Autodesk Inventor part; units mm, degrees
ref_plane "YZ Plane" through (0, 0, 0) normal (1, 0, 0) x (0, 1, 0)
ref_plane "XZ Plane" through (0, 0, 0) normal (0, 1, 0) x (-1, 0, 0)
ref_plane "XY Plane" through (0, 0, 0) normal (0, 0, 1) x (1, 0, 0)
sketch "Sketch1" plane through (0, 0, 0) normal (0, 0, 1) x (1, 0, 0)
  line L0 (-47.9977, 34.7826) -> (52.0023, 34.7826)
  line L1 (52.0023, 34.7826) -> (52.0023, -65.2174)
  line L2 (52.0023, -65.2174) -> (-47.9977, -65.2174)
  line L3 (-47.9977, -65.2174) -> (-47.9977, 34.7826)
  point P0 (0, 0)
  dimension "d0" = 100
  dimension "d1" = 100
  dimension "d2" = 100
extrude "Extrusion1" add sketch "Sketch1" along normal blind 20
sketch "Sketch2" plane through (0, 0, 20) normal (0, 0, 1) x (1, 0, 0)
  line L0 (-22.9977, 9.7826) -> (27.0023, 9.7826)
  line L1 (27.0023, 9.7826) -> (27.0023, -40.2174)
  line L2 (27.0023, -40.2174) -> (-22.9977, -40.2174)
  line L3 (-22.9977, -40.2174) -> (-22.9977, 9.7826)
  line L4 (52.0023, 34.7826) -> (-47.9977, 34.7826)
  line L5 (-47.9977, 34.7826) -> (-47.9977, -65.2174)
  line L6 (-47.9977, -65.2174) -> (52.0023, -65.2174)
  line L7 (52.0023, -65.2174) -> (52.0023, 34.7826)
  point P0 (0, 0)
  dimension "d5" = 25
  dimension "d6" = 25
  dimension "d7" = 25
  dimension "d8" = 25
extrude "Extrusion2" add sketch "Sketch2" along normal blind 100 contours L0 L1 L2 L3
shell "Shell1" thickness 10 removed faces 1 at (-6.331, -6.8841, 120)
sketch "Sketch3" plane through (0, 0, 120) normal (0, 0, 1) x (1, 0, 0)
  line L0 (-22.9977, 9.7826) -> (-22.9977, -40.2174)
  line L1 (27.0023, -40.2174) -> (27.0023, 9.7826)
  line L2 (-22.9977, 9.7826) -> (27.0023, 9.7826)
  line L3 (27.0023, 9.7826) -> (27.0023, -40.2174)
  line L4 (27.0023, -40.2174) -> (-22.9977, -40.2174)
  line L5 (-22.9977, -40.2174) -> (-22.9977, 9.7826)
  point P0 (0, 0)
extrude "Extrusion3" add sketch "Sketch3" along normal blind 13.65
sketch "Sketch4" plane through (0, 0, 133.65) normal (0, 0, 1) x (1, 0, 0)
  line L0 (-22.9977, 9.7826) -> (-4.3577, 9.7826)
  line L1 (-4.3577, 9.7826) -> (-4.3577, -8.8574)
  line L2 (-4.3577, -8.8574) -> (-22.9977, -8.8574)
  line L3 (-22.9977, -8.8574) -> (-22.9977, 9.7826)
  line L4 (27.0023, 9.7826) -> (8.3623, 9.7826)
  line L5 (8.3623, 9.7826) -> (8.3623, -8.8574)
  line L6 (8.3623, -8.8574) -> (27.0023, -8.8574)
  line L7 (27.0023, -8.8574) -> (27.0023, 9.7826)
  line L8 (27.0023, -40.2174) -> (-22.9977, -40.2174)
  line L9 (-22.9977, -40.2174) -> (-4.3577, -40.2174)
  line L10 (-4.3577, -40.2174) -> (-4.3577, -21.5774)
  line L11 (-4.3577, -21.5774) -> (-22.9977, -21.5774)
  line L12 (-22.9977, -21.5774) -> (-22.9977, -40.2174)
  point P0 (0, 0)
  dimension "d14" = 18.64
  dimension "d15" = 18.64
  dimension "d16" = 18.64
  dimension "d17" = 18.64
  dimension "d18" = 18.64
extrude "Extrusion4" add sketch "Sketch4" along normal blind 12.8
sketch "Sketch5" plane through (0, 0, 146.45) normal (0, 0, 1) x (1, 0, 0)
  line L0 (13.3623, 4.7826) -> (22.0023, 4.7826)
  line L1 (22.0023, 4.7826) -> (22.0023, -3.8574)
  line L2 (22.0023, -3.8574) -> (13.3623, -3.8574)
  line L3 (13.3623, -3.8574) -> (13.3623, 4.7826)
  line L4 (-17.9977, 4.7826) -> (-9.3577, 4.7826)
  line L5 (-9.3577, 4.7826) -> (-9.3577, -3.8574)
  line L6 (-9.3577, -3.8574) -> (-17.9977, -3.8574)
  line L7 (-17.9977, -3.8574) -> (-17.9977, 4.7826)
  line L8 (-17.9977, -26.5774) -> (-9.3577, -26.5774)
  line L9 (-9.3577, -26.5774) -> (-9.3577, -35.2174)
  line L10 (-9.3577, -35.2174) -> (-17.9977, -35.2174)
  line L11 (-17.9977, -35.2174) -> (-17.9977, -26.5774)
  line L12 (-4.3577, 9.7826) -> (-22.9977, 9.7826)
  line L13 (-22.9977, 9.7826) -> (-22.9977, -8.8574)
  line L14 (-22.9977, -8.8574) -> (-4.3577, -8.8574)
  line L15 (-4.3577, -8.8574) -> (-4.3577, 9.7826)
  line L16 (27.0023, 9.7826) -> (8.3623, 9.7826)
  line L17 (27.0023, -8.8574) -> (27.0023, 9.7826)
  line L18 (8.3623, 9.7826) -> (8.3623, -8.8574)
  line L19 (-4.3577, -21.5774) -> (-22.9977, -21.5774)
  line L20 (-22.9977, -40.2174) -> (-4.3577, -40.2174)
  point P0 (0, 0)
  dimension "d21" = 5
  dimension "d22" = 5
  dimension "d23" = 5
  dimension "d24" = 5
  dimension "d25" = 5
  dimension "d26" = 5
  dimension "d27" = 5
  dimension "d28" = 5
  dimension "d29" = 5
extrude "Extrusion5" cut sketch "Sketch5" against normal blind 15 contours L0 L1 L2 L3 | L4 L5 L6 L7 | L8 L9 L10 L11
equation "\"d1\" = d0"
equation "\"d6\" = d5"
equation "\"d7\" = d5"
equation "\"d8\" = d5"
equation "\"d15\" = d14"
equation "\"d16\" = d14"
equation "\"d18\" = d14"
equation "\"d22\" = d21"
equation "\"d23\" = d21"
equation "\"d24\" = d21"
equation "\"d26\" = d21"
equation "\"d27\" = d21"
equation "\"d28\" = d21"
equation "\"d29\" = d21"
properties part number "final_beam_cube"
Input: part model. Units: mm. Frame: model coordinates. A direction names the side the tool comes from. Coordinates: 2 decimals unless noted, no trailing zeros. Loops run counter-clockwise (first coordinate to the right, second up) from the corner with the lowest first, then second, coordinate; pieces in that order, holes last. Notation, with made-up numbers: (89, 46) -> (144, 46) arc R28 cw to (144, 67) -> close; hole circle Ø6 at (46, 55). An arc over 180 degrees is marked (long way). Use a Markdown table: item, result.
1) Cut plane C-C (x = -16). Return the cut outline in (y, z).
Results found:
| item | result |
|---|---|
| outline | (-65.22, 0) -> (34.78, 0) -> (34.78, 20) -> (9.78, 20) -> (9.78, 146.45) -> (4.78, 146.45) -> (4.78, 131.45) -> (-3.86, 131.45) -> (-3.86, 146.45) -> (-8.86, 146.45) -> (-8.86, 133.65) -> (-21.58, 133.65) -> (-21.58, 146.45) -> (-26.58, 146.45) -> (-26.58, 131.45) -> (-35.22, 131.45) -> (-35.22, 146.45) -> (-40.22, 146.45) -> (-40.22, 20) -> (-65.22, 20) -> close |
2) Pull-direction query (Y, two-part tool) for faces 1 (the flat face through (-17.998, 0, 139)), 2 (the flat face through (18, -8.857, 140)), 3 (the flat face through (-8, -31, 146.45)); classes: released by +Y, released by -Y, zero draft, split by the parting line, or undercut.
Results found:
| item | result |
|---|---|
| face 1 | undercut |
| face 2 | released by -Y |
| face 3 | zero draft |
3) Material intervals for line 1 along X through (y, z) = (-18, 88); line 2 along X through (y, z) = (-27.5, 133); line 3 along Y through (x, z) = (8, 44), sorted ascending. Write a range as from..to.
Results found:
| item | result |
|---|---|
| line 1 | x = -23..-13, 17..27 |
| line 2 | x = -23..-18, -9.36..27 |
| line 3 | y = -40.22..-30.22, -0.22..9.78 |
4) Cut plane D-D (z = 70). Return the cut outline in (x, y).
Results found:
| item | result |
|---|---|
| outline | (-23, -40.22) -> (27, -40.22) -> (27, 9.78) -> (-23, 9.78) -> close; hole (-13, -30.22) -> (17, -30.22) -> (17, -0.22) -> (-13, -0.22) -> close |
5) Cut plane A-A (y = -11). Return the cut outline in (x, z).
Results found:
| item | result |
|---|---|
| outline | (-48, 0) -> (52, 0) -> (52, 20) -> (27, 20) -> (27, 133.65) -> (-23, 133.65) -> (-23, 20) -> (-48, 20) -> close; hole (-13, 10) -> (17, 10) -> (17, 120) -> (-13, 120) -> close |
6) Cut plane B-B (z = 17.5). Return the cut outline in (x, y).
Results found:
| item | result |
|---|---|
| outline | (-48, -65.22) -> (52, -65.22) -> (52, 34.78) -> (-48, 34.78) -> close; hole (-13, -30.22) -> (17, -30.22) -> (17, -0.22) -> (-13, -0.22) -> close |
7) Access query for faces 4 (the flat face through (18, 1, 131.45)), 5 (the flat face through (2, -30.217, 64)), 6 (the flat face through (-4.358, 1, 140)), 7 (the flat face through (2, -40.217, 82)). Directions: +Z, -Z, +X, -X, +Y, -Y. A direction counts if a zero-diameter tool reaches every point of the face in a straight line with its end or side. Return the directions, or none.
Results found:
| item | result |
|---|---|
| face 4 | +Z |
| face 5 | none |
| face 6 | +Z, +Y, -Y |
| face 7 | +Z, +X, -X, -Y |
8) Contact query for flat-ended pins moving along their axis: pin 1 (1.5 mm diameter, centred on x = -2.5, z = 55.5, fed in from +Y); pin 2 (9.5 mm diameter, centred on y = -0.5, z = 135.5, fed in from +X); pin 3 (9.5 mm diameter, centred on x = -15.5, z = 137.5, fed in from -Y). Output: stop coordinate, or through.
Results found:
| item | result |
|---|---|
| pin 1 | stops at y = 9.78 |
| pin 2 | stops at x = 27 |
| pin 3 | stops at y = -40.22 |
